Design review of the part built by this model. Coordinates are the model's own, in mm. A direction names the side the tool comes from. Give positions to 0.01 mm unless a question says otherwise; leave off trailing zeros. Loops run counter-clockwise (first coordinate to the right, second up) from the corner with the lowest first, then second, coordinate; pieces in that order, holes last. Notation, with made-up numbers: M -19.5,-10 L 3.5,-10 A22 cw 3.5,17 Z; hole C 79,-38 d10. An arc over 180 degrees is marked long. Use a Markdown table: item, result. Add a question column.
(1) Add section D-D, the plane x = 8.5. Give the boundary of the cut face in (y, z), then the cut area to 3 significant figures.
(2) Add section C-C, the plane y = 1.55. State how many separate pieces and enclosed holes the cut face has, then the cut area to 3 significant figures.
(3) Add section A-A, the plane z = 0. Give the boundary of the cut face in (x, y).
(4) For faces 1 (the face through (11, 0, -1)), 2 (the face through (25, 2, 9.5)), list the 3-axis set-ups (+Z, -Z, +X, -X, +Y, -Y) from which the entire face can be reached by the end or side of a thin tool; tool diameter is ignored.
(5) Add section B-B, the plane z = 6. Give the boundary of the cut face in (x, y), then the cut area to 4 significant figures.
(6) Insertion check: pin 1 Ø1 at (y, z) = (0.5, -2.5) entering from -X; pin 2 Ø1.5 at (y, z) = (2, -3.5) entering from -X; pin 3 Ø1.5 at (x, y) = (23.5, 1) entering from -Z. Each pin has a flat end and moves straight along its axis. Give the tip position at first contact, or say it passes through.
(7) Draft analysis for pull direction Z (two halves, no side actions). For faces 3 (the face through (3.28, 1.48, -7.4)), 4 (the face through (11, 3, -1)), 5 (the face through (25, 2, 6.5)), state which applies: pulls with the +Z half, pulls with the -Z half, needs draft (parallel to the pull), parting line crosses it, or undercut.
(8) For probe 1 along X at (y, z) = (1, -0.5); probe 2 along Z at (x, y) = (22.5, 0.5); probe 3 along X at (y, z) = (2.75, -1), list the stretches that pass through material, from the lowest coordinate up.
```python
from build123d import *

# Parameters (mm, degrees)
SKETCH1_R           = 2.1
BOSS_EXTRUDE1_DEPTH = 3
FILLET1_R           = 5
SKETCH2_W           = 10
SKETCH2_H           = 3
CUT_EXTRUDE1_DEPTH  = 3


with BuildPart() as part:
    # Sketch1 → Boss-Extrude1 (new body)
    with BuildSketch(Plane(origin=(0, 0, 0), x_dir=(1, 0, 0), z_dir=(0, 1, 0))):
        with BuildLine():
            Line((0, -11.456439237), (0, -12.5))
            Line((0, -12.5), (30, -12.5))
            Line((30, -12.5), (30, -4.955880937))
            ThreePointArc((30, -4.955880937), (29.758770483, -3.587800364), (29.064177772, -2.384730498))
            Line((29.064177772, -2.384730498), (25.555494336, 1.796755592))
            ThreePointArc((25.555494336, 1.796755592), (24.386056013, 5.068955923), (25.631429931, 8.313015849))
            ThreePointArc((25.631429931, 8.313015849), (23.39515563, 19.95401875), (12.677699795, 14.889434685))
            ThreePointArc((12.677699795, 14.889434685), (11.918282987, 13.141523465), (10.560020318, 11.804725034))
            Line((10.560020318, 11.804725034), (5.017813295, 8.128440794))
            ThreePointArc((5.017813295, 8.128440794), (3.258028142, 7.396960283), (1.352375582, 7.377064476))
            ThreePointArc((1.352375582, 7.377064476), (-7.172928544, 2.190683933), (-3, -6.873863542))
            ThreePointArc((-3, -6.873863542), (-0.816699867, -8.71782645), (0, -11.456439237))
        make_face()
        with Locations(Location((0, 0, 0), (0, 0, 270))):
            Circle(SKETCH1_R, mode=Mode.SUBTRACT)
        with Locations(Location((20, 13.266499161, 0), (0, 0, 270))):
            Circle(SKETCH1_R, mode=Mode.SUBTRACT)
    extrude(amount=BOSS_EXTRUDE1_DEPTH)

    # Fillet1
    fillet1_edges = [part.edges().sort_by_distance(p)[0] for p in [
        (0, 1.5, 12.5),
    ]]
    fillet(fillet1_edges, radius=FILLET1_R)

    # Sketch2 → Cut-Extrude1 (cut)
    with BuildSketch(Plane(origin=(0, 3, 0), x_dir=(1, 0, 0), z_dir=(0, 1, 0))):
        with Locations((25, -8)):
            Rectangle(SKETCH2_W, SKETCH2_H)
    extrude(amount=-CUT_EXTRUDE1_DEPTH, mode=Mode.SUBTRACT)


solid = part.part
```
Established:
| question | item | result |
|---|---|---|
| 1 | outline | M 0,-10.44 L 3,-10.44 L 3,12.5 L 0,12.5 Z |
| 1 | area | 68.8 mm^2 |
| 2 | separate pieces | 1 |
| 2 | enclosed holes | 2 |
| 2 | area | 782 mm^2 |
| 3 | outline | M -7.5,0 L -2.1,0 L -2.1,3 L -7.5,3 Z; M 2.1,0 L 27.06,0 L 27.06,3 L 2.1,3 Z |
| 4 | face 1 | +Z, -Z, +X, -X, -Y |
| 4 | face 2 | +X, +Y, -Y |
| 5 | outline | M -4.5,0 L 30,0 L 30,3 L -4.5,3 Z |
| 5 | area | 103.5 mm^2 |
| 6 | pin 1 | x = -7.23 |
| 6 | pin 2 | x = -6.98 |
| 6 | pin 3 | z = -20.24 |
| 7 | face 3 | pulls with the -Z half |
| 7 | face 4 | needs draft |
| 7 | face 5 | undercut |
| 8 | probe 1 | -7.48 to -2.04, 2.04 to 26.64 |
| 8 | probe 2 | -20.34 to 6.5, 9.5 to 12.5 |
| 8 | probe 3 | -7.43 to -1.85, 1.85 to 26.22 |
